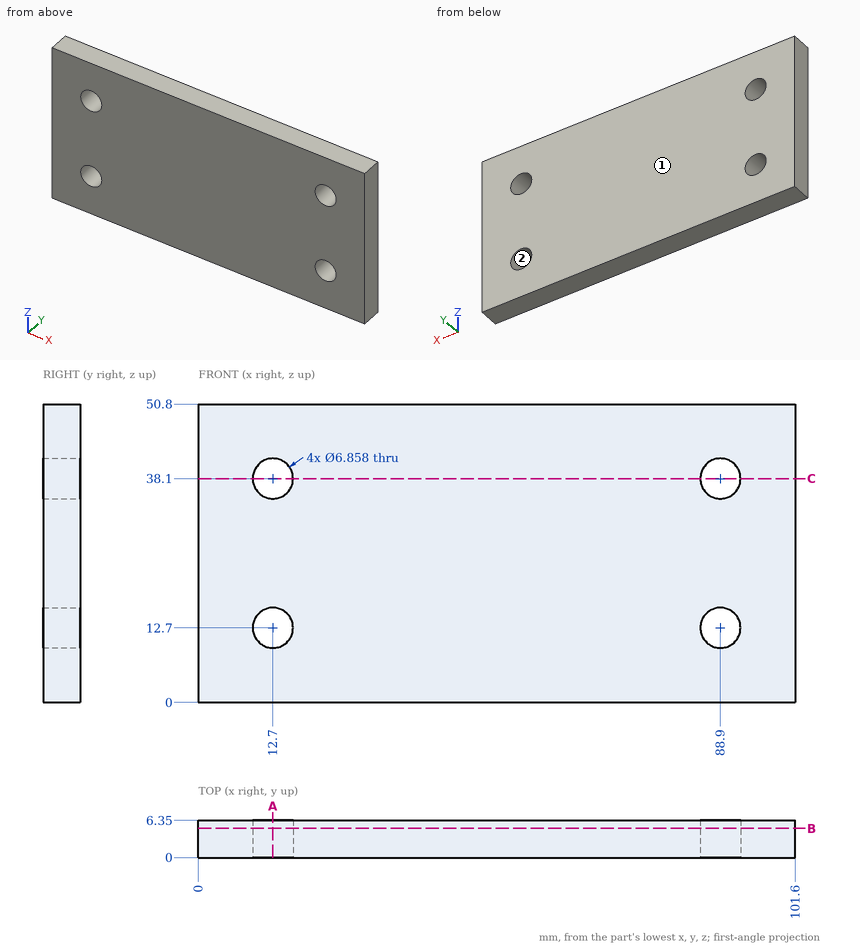
Geometry: see drawing. Coordinates: mm, zero at the bounding-box minimum. Give positions to 0.01 mm unless a question says otherwise; leave off trailing zeros. Order: outer loops, then holes, each group sorted by start corner. A loop starts at its lowest first (then second) coordinate and runs counter-clockwise, first axis right, second up.
Q1. Section B-B on y = 5. Output: boundary loops of the cut face in (x, z).
Checked values:
outline: (0, 0) - (101.6, 0) - (101.6, 50.8) - (0, 50.8) - close; hole circle Ø6.86 at (12.7, 12.7); hole circle Ø6.86 at (12.7, 38.1); hole circle Ø6.86 at (88.9, 12.7); hole circle Ø6.86 at (88.9, 38.1)
Q2. Contact query for flat-ended pins moving along their axis: pin 1 Ø5.5 at (x, z) = (12.7, 38.1) entering from +Y; pin 2 Ø1.5 at (y, z) = (5, 9) entering from -X. Output: stop coordinate, or through.
Checked values:
pin 1: passes through
pin 2: stops at x = 0
Q3. Ray query, probe 1 along X at (y, z) = (2.5, 12.7); probe 2 along Z at (x, y) = (88.9, 4); probe 3 along Z at (x, y) = (88, 3.75). Return the intervals inside material, ascending.
Checked values:
probe 1: x = 0 to 9.27, 16.13 to 85.47, 92.33 to 101.6
probe 2: z = 0 to 9.27, 16.13 to 34.67, 41.53 to 50.8
probe 3: z = 0 to 9.39, 16.01 to 34.79, 41.41 to 50.8
Q4. Section A-A on x = 12.7. Output: boundary loops of the cut face in (y, z).
Checked values:
outline: (0, 0) - (6.35, 0) - (6.35, 9.27) - (0, 9.27) - close; (0, 16.13) - (6.35, 16.13) - (6.35, 34.67) - (0, 34.67) - close; (0, 41.53) - (6.35, 41.53) - (6.35, 50.8) - (0, 50.8) - close
Q5. Draft query along Z for the marked faces 1 and 2. Return one class per face: +Z half, -Z half, draft (parallel to the pull), parting line (faces both ways), or undercut.
Checked values:
face 1: draft
face 2: undercut
Q6. Section C-C on z = 38.1. Output: boundary loops of the cut face in (x, y).
Checked values:
outline: (0, 0) - (9.27, 0) - (9.27, 6.35) - (0, 6.35) - close; (16.13, 0) - (85.47, 0) - (85.47, 6.35) - (16.13, 6.35) - close; (92.33, 0) - (101.6, 0) - (101.6, 6.35) - (92.33, 6.35) - close
